Part model, mm, in its own coordinate system. A direction names the side the tool comes from. Give positions to 0.01 mm unless a question says otherwise; leave off trailing zeros. Loops run counter-clockwise (first coordinate to the right, second up) from the corner with the lowest first, then second, coordinate; pieces in that order, holes last. Notation, with made-up numbers: M 58.5,76.5 L 92.5,76.5 A21 ccw 92.5,114.5 Z; hole C -33,-39 d5. An arc over 180 degrees is marked long. Answer in a Markdown table with one row per item.
Autodesk Inventor part; units mm, degrees
ref_plane "YZ Plane" through (0, 0, 0) normal (1, 0, 0) x (0, 1, 0)
ref_plane "XZ Plane" through (0, 0, 0) normal (0, 1, 0) x (-1, 0, 0)
ref_plane "XY Plane" through (0, 0, 0) normal (0, 0, 1) x (1, 0, 0)
sketch "Sketch1" plane through (0, 0, 0) normal (0, 1, 0) x (-1, 0, 0)
  circle A0 centre (0, 0) radius 19.05
  dimension "d0" = 38.1
extrude "Extrusion1" add sketch "Sketch1" along normal blind 3.175
sketch "Sketch2" plane through (0, 3.175, 0) normal (0, 1, 0) x (1, 0, 0)
  circle A0 centre (0, 0) radius 6.35
  dimension "d3" = 12.7
extrude "Extrusion2" add sketch "Sketch2" along normal blind 6.35
sketch "Sketch3" plane through (0, 9.525, 0) normal (0, 1, 0) x (1, 0, 0)
  circle A0 centre (0, 0) radius 14.2875
  dimension "d6" = 28.575
extrude "Extrusion3" add sketch "Sketch3" along normal blind 6.35
chamfer "Chamfer1" distance 7.9375 angle 30 1 edges at (-14.2875, 9.525, 0) measured on face at (11.4418, 9.525, 1.6463)
chamfer "Chamfer2" distance 3.175 angle 30 1 edges at (19.05, 3.175, 0) measured on face at (-14.6321, 3.175, -1.5197)
sketch "Sketch4" plane through (0, 15.875, 0) normal (0, 1, 0) x (1, 0, 0)
  circle A0 centre (-10.16, 0) radius 1.27
  circle A1 centre (10.16, 0) radius 1.27
  circle A2 centre (0, 0) radius 6.35
  dimension "d15" = 2.54
  dimension "d16" = 10.16
  dimension "d17" = 10.16
extrude "Extrusion4" cut sketch "Sketch4" against normal up to surface (12.7 mm away) contours A0 | A1
sketch "Sketch5" plane through (0, 15.875, 0) normal (0, 1, 0) x (1, 0, 0)
  circle A0 centre (0, 0) radius 3
  line L0 (-1.6583, -2.5) -> (1.6583, -2.5)
  point P0 (0, 3)
  dimension "d20" = 6
  dimension "d21" = 5.5
extrude "Extrusion5" cut sketch "Sketch5" against normal through all contours A0 L0 picked at (0.1141, -0.6732)
properties part number "Pulley_3DPrint"
(1) Pull direction Y, two halves, no side cores. Call faces 6 (the face through (3.48, 3.06, 15.69)), 7 (the face through (-8.99, 14.01, 0.49)), 8 (the face through (-1.38, 6.31, -6.2)), 9 (the face through (6.5, 9.8, -2.1)): +Y half, -Y half, draft (parallel to the pull), parting line (faces both ways), or undercut.
Recorded:
| item | result |
|---|---|
| face 6 | +Y half |
| face 7 | draft |
| face 8 | undercut |
| face 9 | undercut |
(2) Saw through at C-C (z = 0). Give the number of separate pieces and of enclosed holes in the cut face, plus the area to 3 significant figures.
Recorded:
| item | result |
|---|---|
| separate pieces | 4 |
| enclosed holes | 0 |
| area | 225 mm^2 |
(3) Which spindle directions (+Z, -Z, +X, -X, +Y, -Y) get a long thin tool onto all of the face, cutting with end or side? Do faces 1 (the face through (-7, 3.175, 0)), 2 (the face through (-4, 0, 0)), 3 (the face through (0, 15.875, 3)), 4 (the face through (0, 8, 2.5)), 5 (the face through (8.89, 14.01, -0.06)). Say none if no direction does.
Recorded:
| item | result |
|---|---|
| face 1 | none |
| face 2 | +Z, -Z, +X, -X, -Y |
| face 3 | +Z, -Z, +X, -X, +Y |
| face 4 | +Y, -Y |
| face 5 | +Y |
(4) Saw through at B-B (y = 14.75). Write the cut outline in (x, z) (1 decimal).
Recorded:
| item | result |
|---|---|
| outline | C 0,0 d28.6; hole C -10.2,0 d2.5; hole M -1.7,2.5 A3 ccw long 1.7,2.5 Z; hole C 10.2,0 d2.5 |
(5) Pin check, flat tips, straight feed: pin 1 Ø4 at (y, z) = (4, 3) entering from -X; pin 2 Ø1 at (x, y) = (-0.5, 6.5) entering from -Z; pin 3 Ø4 at (y, z) = (6, 2.5) entering from +X. Stop position of each tip, or through.
Recorded:
| item | result |
|---|---|
| pin 1 | stops at x = -17.67 |
| pin 2 | stops at z = -6.35 |
| pin 3 | stops at x = 6.33 |
(6) Drill centre lines: line 1 along X through (y, z) = (14.2, 0); line 2 along Y through (x, z) = (15.5, 0) (3 decimals); line 3 along Z through (x, y) = (0, 8). Where is each one in solid material? Low to high.
Recorded:
| item | result |
|---|---|
| line 1 | x = -14.29 to -11.43, -8.89 to -3, 3 to 8.89, 11.43 to 14.29 |
| line 2 | y = 0 to 3.175 |
| line 3 | z = -6.35 to -3, 2.5 to 6.35 |
